The listing builds one solid part. Answer for the finished solid, in the listing's coordinates (mm). Coordinates: 2 decimals unless noted, no trailing zeros. Order: outer loops, then holes, each group sorted by start corner. A loop starts at its lowest first (then second) coordinate and runs counter-clockwise, first axis right, second up. Notation, with made-up numbers: (89, -2) -> (100, -2) arc R26 cw to (100, 18) -> close; hole circle Ø8 at (42, 0.5). An arc over 180 degrees is marked (long way). Answer in a Markdown table with one row per item.
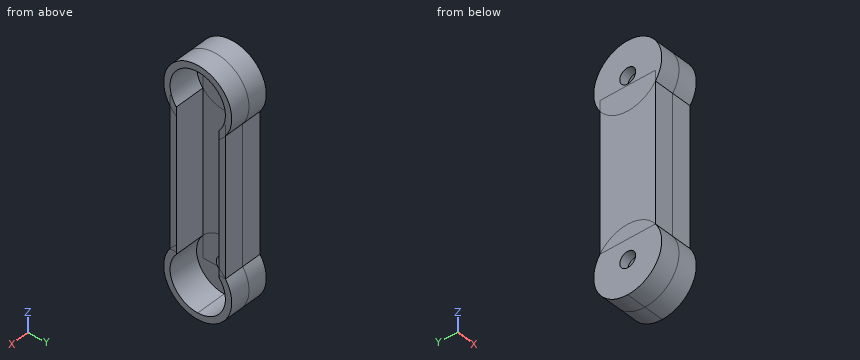
```python
from build123d import *

# Parameters (mm, degrees)
CROQUIS1_R              = 5
SALIENTE_EXTRUIR1_DEPTH = 12.5
CORTAR_EXTRUIR1_START   = -19.2
CROQUIS2_R              = 5
CORTAR_EXTRUIR1_DEPTH   = 19.2


with BuildPart() as part:
    # Croquis1 → Saliente-Extruir1 (new, symmetric)
    # profile 1 of 5: a face of its own
    with BuildSketch(Plane(origin=(0, 0, 0), x_dir=(0, 0, -1), z_dir=(1, 0, 0))):
        with BuildLine():
            Line((-46.862494928, -17.533403612), (-46.862494928, 17.533403612))
            Line((-46.862494928, 17.533403612), (-40.251383817, 17.533403612))
            ThreePointArc((-40.251383817, 17.533403612), (-74.194444444, 0), (-40.251383817, -17.533403612))
            Line((-40.251383817, -17.533403612), (-46.862494928, -17.533403612))
        make_face()
        with Locations((-52.694444444, 0)):
            Circle(CROQUIS1_R, mode=Mode.SUBTRACT)
    # profile 2 of 5: a face of its own
    with BuildSketch(Plane(origin=(0, 0, 0), x_dir=(0, 0, -1), z_dir=(1, 0, 0))):
        with BuildLine():
            Line((-40.251383817, 17.533403612), (-46.862494928, 17.533403612))
            Line((-46.862494928, 17.533403612), (-46.862494928, -17.533403612))
            Line((-46.862494928, -17.533403612), (-40.251383817, -17.533403612))
            ThreePointArc((-40.251383817, -17.533403612), (-33.592405241, -9.867223432), (-31.194444444, 0))
            ThreePointArc((-31.194444444, 0), (-33.592405241, 9.867223432), (-40.251383817, 17.533403612))
        make_face()
    # profile 3 of 5: a face of its own
    with BuildSketch(Plane(origin=(0, 0, 0), x_dir=(0, 0, -1), z_dir=(1, 0, 0))):
        with BuildLine():
            Line((46.862494928, 17.533403612), (-40.251383817, 17.533403612))
            ThreePointArc((-40.251383817, 17.533403612), (-33.592405241, 9.867223432), (-31.194444444, 0))
            ThreePointArc((-31.194444444, 0), (-33.592405241, -9.867223432), (-40.251383817, -17.533403612))
            Line((-40.251383817, -17.533403612), (46.862494928, -17.533403612))
            ThreePointArc((46.862494928, -17.533403612), (37.805555556, 0), (46.862494928, 17.533403612))
        make_face()
    # profile 4 of 5: a face of its own
    with BuildSketch(Plane(origin=(0, 0, 0), x_dir=(0, 0, -1), z_dir=(1, 0, 0))):
        with BuildLine():
            Line((46.862494928, -17.533403612), (46.862494928, 17.533403612))
            ThreePointArc((46.862494928, 17.533403612), (37.805555556, 0), (46.862494928, -17.533403612))
        make_face()
    # profile 5 of 5: a face of its own
    with BuildSketch(Plane(origin=(0, 0, 0), x_dir=(0, 0, -1), z_dir=(1, 0, 0))):
        with BuildLine():
            ThreePointArc((80.805555556, 0), (69.172778987, 19.102039204), (46.862494928, 17.533403612))
            Line((46.862494928, 17.533403612), (46.862494928, -17.533403612))
            ThreePointArc((46.862494928, -17.533403612), (69.172778987, -19.102039204), (80.805555556, 0))
        make_face()
        with Locations((59.305555556, 0)):
            Circle(CROQUIS1_R, mode=Mode.SUBTRACT)
    extrude(amount=SALIENTE_EXTRUIR1_DEPTH, both=True)

    # Croquis2 → Cortar-Extruir1 (cut)
    # profile 1 of 7: a face of its own
    with BuildSketch(Plane(origin=(12.5, 0, 0), x_dir=(0, 0, -1), z_dir=(1, 0, 0)).offset(CORTAR_EXTRUIR1_START)):
        with BuildLine():
            Line((-61.940275078, -13.533403612), (-61.940275078, 13.533403612))
            Line((-61.940275078, 13.533403612), (-41.599536302, 13.533403612))
            ThreePointArc((-41.599536302, 13.533403612), (-70.194444444, 0), (-41.599536302, -13.533403612))
            Line((-41.599536302, -13.533403612), (-61.940275078, -13.533403612))
        make_face()
    # profile 2 of 7: a face of its own
    with BuildSketch(Plane(origin=(12.5, 0, 0), x_dir=(0, 0, -1), z_dir=(1, 0, 0)).offset(CORTAR_EXTRUIR1_START)):
        with BuildLine():
            Line((-41.599536302, 13.533403612), (-61.940275078, 13.533403612))
            Line((-61.940275078, 13.533403612), (-61.940275078, -13.533403612))
            Line((-61.940275078, -13.533403612), (-41.599536302, -13.533403612))
            ThreePointArc((-41.599536302, -13.533403612), (-36.876560697, -7.486291055), (-35.194444444, 0))
            ThreePointArc((-35.194444444, 0), (-36.876560697, 7.486291055), (-41.599536302, 13.533403612))
        make_face()
        with Locations((-52.694444444, 0)):
            Circle(CROQUIS2_R, mode=Mode.SUBTRACT)
    # profile 3 of 7: a face of its own
    with BuildSketch(Plane(origin=(12.5, 0, 0), x_dir=(0, 0, -1), z_dir=(1, 0, 0)).offset(CORTAR_EXTRUIR1_START)):
        with BuildLine():
            Line((48.210647414, 13.533403612), (-41.599536302, 13.533403612))
            ThreePointArc((-41.599536302, 13.533403612), (-36.876560697, 7.486291055), (-35.194444444, 0))
            ThreePointArc((-35.194444444, 0), (-36.876560697, -7.486291055), (-41.599536302, -13.533403612))
            Line((-41.599536302, -13.533403612), (48.210647414, -13.533403612))
            ThreePointArc((48.210647414, -13.533403612), (41.805555556, 0), (48.210647414, 13.533403612))
        make_face()
    # profile 4 of 7: a face of its own
    with BuildSketch(Plane(origin=(12.5, 0, 0), x_dir=(0, 0, -1), z_dir=(1, 0, 0)).offset(CORTAR_EXTRUIR1_START)):
        with BuildLine():
            ThreePointArc((76.805555556, 0), (66.79184661, 15.817883747), (48.210647414, 13.533403612))
            Line((48.210647414, 13.533403612), (61.940275078, 13.533403612))
            Line((61.940275078, 13.533403612), (61.940275078, 4.249500328))
            ThreePointArc((61.940275078, 4.249500328), (63.67439966, 2.431707465), (64.305555556, 0))
            ThreePointArc((64.305555556, 0), (63.67439966, -2.431707465), (61.940275078, -4.249500328))
            Line((61.940275078, -4.249500328), (61.940275078, -13.533403612))
            Line((61.940275078, -13.533403612), (48.210647414, -13.533403612))
            ThreePointArc((48.210647414, -13.533403612), (66.79184661, -15.817883747), (76.805555556, 0))
        make_face()
    # profile 5 of 7: a face of its own
    with BuildSketch(Plane(origin=(12.5, 0, 0), x_dir=(0, 0, -1), z_dir=(1, 0, 0)).offset(CORTAR_EXTRUIR1_START)):
        with BuildLine():
            Line((61.940275078, 13.533403612), (48.210647414, 13.533403612))
            ThreePointArc((48.210647414, 13.533403612), (41.805555556, 0), (48.210647414, -13.533403612))
            Line((48.210647414, -13.533403612), (61.940275078, -13.533403612))
            Line((61.940275078, -13.533403612), (61.940275078, -4.249500328))
            ThreePointArc((61.940275078, -4.249500328), (54.305555556, 0), (61.940275078, 4.249500328))
            Line((61.940275078, 4.249500328), (61.940275078, 13.533403612))
        make_face()
    # profile 6 of 7: a face of its own
    with BuildSketch(Plane(origin=(12.5, 0, 0), x_dir=(0, 0, -1), z_dir=(1, 0, 0)).offset(CORTAR_EXTRUIR1_START)):
        with BuildLine():
            ThreePointArc((76.805555556, 0), (66.79184661, 15.817883747), (48.210647414, 13.533403612))
            Line((48.210647414, 13.533403612), (61.940275078, 13.533403612))
            Line((61.940275078, 13.533403612), (61.940275078, 4.249500328))
            ThreePointArc((61.940275078, 4.249500328), (63.67439966, 2.431707465), (64.305555556, 0))
            ThreePointArc((64.305555556, 0), (63.67439966, -2.431707465), (61.940275078, -4.249500328))
            Line((61.940275078, -4.249500328), (61.940275078, -13.533403612))
            Line((61.940275078, -13.533403612), (48.210647414, -13.533403612))
            ThreePointArc((48.210647414, -13.533403612), (66.79184661, -15.817883747), (76.805555556, 0))
        make_face()
    # profile 7 of 7: a face of its own
    with BuildSketch(Plane(origin=(12.5, 0, 0), x_dir=(0, 0, -1), z_dir=(1, 0, 0)).offset(CORTAR_EXTRUIR1_START)):
        with BuildLine():
            Line((61.940275078, 13.533403612), (48.210647414, 13.533403612))
            ThreePointArc((48.210647414, 13.533403612), (41.805555556, 0), (48.210647414, -13.533403612))
            Line((48.210647414, -13.533403612), (61.940275078, -13.533403612))
            Line((61.940275078, -13.533403612), (61.940275078, -4.249500328))
            ThreePointArc((61.940275078, -4.249500328), (54.305555556, 0), (61.940275078, 4.249500328))
            Line((61.940275078, 4.249500328), (61.940275078, 13.533403612))
        make_face()
    extrude(amount=CORTAR_EXTRUIR1_DEPTH, mode=Mode.SUBTRACT)


solid = part.part
```
(1) Flat-ended cylindrical pins translate along their axes: pin 1 (16 mm diameter, centred on y = -2.5, z = -48.5, fed in from +X); pin 2 (2 mm diameter, centred on x = 7.5, y = -9.5, fed in from -Z); pin 3 (6 mm diameter, centred on x = 4, z = 4.5, fed in from +Y). Find the tip coordinate at first contact, or state that the pin passes through.
Check values:
| item | result |
|---|---|
| pin 1 | x = -6.7 |
| pin 2 | z = -79.05 |
| pin 3 | y = 17.53 |
(2) A cutting plane is placed at A-A, the plane x = -10.5. Determine the outline of the cut face in (y, z), then the cut area to 3 significant figures.
Check values:
| item | result |
|---|---|
| outline | (-17.53, -46.86) arc R21.5 ccw (long way) to (17.53, -46.86) -> (17.53, 40.25) arc R21.5 ccw (long way) to (-17.53, 40.25) -> close; hole circle Ø10 at (0, -59.31); hole circle Ø10 at (0, 52.69) |
| area | 5,360 mm² |
(3) Find the intervals of material crossed by line 1 along Y through (x, z) = (8.75, 5.5); line 2 along X through (y, z) = (-7, -53); line 3 along Z through (x, y) = (-2, -12), in increasing order. Write a range as from..to.
Check values:
| item | result |
|---|---|
| line 1 | -17.53..-13.53, 13.53..17.53 |
| line 2 | -12.5..-6.7 |
| line 3 | -77.15..-72.04, 65.43..70.53 |
(4) A cutting plane is placed at B-B, the plane z = 11. Determine the outline of the cut face in (x, y), then the cut area to 3 significant figures.
Check values:
| item | result |
|---|---|
| outline | (-12.5, -17.53) -> (12.5, -17.53) -> (12.5, -13.53) -> (-6.7, -13.53) -> (-6.7, 13.53) -> (12.5, 13.53) -> (12.5, 17.53) -> (-12.5, 17.53) -> close |
| area | 357 mm² |
(5) A cutting plane is placed at D-D, the plane y = -2. Determine the outline of the cut face in (x, z).
Check values:
| item | result |
|---|---|
| outline | (-12.5, -80.71) -> (12.5, -80.71) -> (12.5, -76.69) -> (-6.7, -76.69) -> (-6.7, -63.89) -> (-12.5, -63.89) -> close; (-12.5, -54.72) -> (-6.7, -54.72) -> (-6.7, 48.11) -> (-12.5, 48.11) -> close; (-12.5, 57.28) -> (-6.7, 57.28) -> (-6.7, 70.08) -> (12.5, 70.08) -> (12.5, 74.1) -> (-12.5, 74.1) -> close |
(6) A cutting plane is placed at C-C, the plane x = 8.25. Determine the outline of the cut face in (y, z).
Check values:
| item | result |
|---|---|
| outline | (-17.53, -46.86) arc R21.5 ccw (long way) to (17.53, -46.86) -> (17.53, 40.25) arc R21.5 ccw (long way) to (-17.53, 40.25) -> close; hole (-13.53, -48.21) arc R17.5 ccw (long way) to (13.53, -48.21) -> (13.53, 41.6) arc R17.5 ccw (long way) to (-13.53, 41.6) -> close |
